```python
from build123d import *

# Parameters (mm, degrees)
F0_R            = 17.8
F0_R_2          = 7.6
F0_R_3          = 1.75
F1_DEPTH        = 10.7
F2_DEPTH        = 9.7
F2_COPIES_COUNT = 10
F3_DEPTH        = 10.7
F3_COPIES_COUNT = 10


# Not quite as in the source:
# - a pattern or mirror of a feature is missing from the dataset's text; its kind, count and spacing are read off the source's solid


with BuildPart() as f1:
    # F0 (on Top) → F1 (new body)
    with BuildSketch(Plane.XY):
        Circle(F0_R)
        Circle(F0_R_2, mode=Mode.SUBTRACT)
        with BuildLine():
            ThreePointArc((14.45, 2.5588083164), (15.4418059742, 1.4465476141), (15.8, 0))
            ThreePointArc((15.8, 0), (15.4418059742, -1.4465476141), (14.45, -2.5588083164))
            Line((14.45, -2.5588083164), (14.45, -3.5))
            Line((14.45, -3.5), (10.95, -3.5))
            Line((10.95, -3.5), (10.95, -2.5588083164))
            ThreePointArc((10.95, -2.5588083164), (9.6, 0), (10.95, 2.5588083164))
            Line((10.95, 2.5588083164), (10.95, 3.5))
            Line((10.95, 3.5), (14.45, 3.5))
            Line((14.45, 3.5), (14.45, 2.5588083164))
        make_face(mode=Mode.SUBTRACT)
        with BuildLine():
            ThreePointArc((14.45, -2.5588083164), (15.4418059742, -1.4465476141), (15.8, 0))
            ThreePointArc((15.8, 0), (15.4418059742, 1.4465476141), (14.45, 2.5588083164))
            ThreePointArc((14.45, 2.5588083164), (12.7, 3.1), (10.95, 2.5588083164))
            ThreePointArc((10.95, 2.5588083164), (9.6, 0), (10.95, -2.5588083164))
            ThreePointArc((10.95, -2.5588083164), (12.7, -3.1), (14.45, -2.5588083164))
        make_face()
        with Locations((12.7, 0)):
            Circle(F0_R_3, mode=Mode.SUBTRACT)
        with Locations((12.7, 0)):
            Circle(F0_R_3)
        with BuildLine():
            Line((14.45, -3.5), (14.45, -2.5588083164))
            ThreePointArc((14.45, -2.5588083164), (12.7, -3.1), (10.95, -2.5588083164))
            Line((10.95, -2.5588083164), (10.95, -3.5))
            Line((10.95, -3.5), (14.45, -3.5))
        make_face()
        with BuildLine():
            ThreePointArc((10.95, 2.5588083164), (12.7, 3.1), (14.45, 2.5588083164))
            Line((14.45, 2.5588083164), (14.45, 3.5))
            Line((14.45, 3.5), (10.95, 3.5))
            Line((10.95, 3.5), (10.95, 2.5588083164))
        make_face()
    extrude(amount=F1_DEPTH)

    # F0 (on Top) → F2 (cut)
    with BuildSketch(Plane.XY):
        with BuildLine():
            ThreePointArc((14.45, -2.5588083164), (15.4418059742, -1.4465476141), (15.8, 0))
            ThreePointArc((15.8, 0), (15.4418059742, 1.4465476141), (14.45, 2.5588083164))
            ThreePointArc((14.45, 2.5588083164), (12.7, 3.1), (10.95, 2.5588083164))
            ThreePointArc((10.95, 2.5588083164), (9.6, 0), (10.95, -2.5588083164))
            ThreePointArc((10.95, -2.5588083164), (12.7, -3.1), (14.45, -2.5588083164))
        make_face()
        with Locations((12.7, 0)):
            Circle(F0_R_3, mode=Mode.SUBTRACT)
        with Locations((12.7, 0)):
            Circle(F0_R_3)
    f2 = extrude(amount=F2_DEPTH, mode=Mode.SUBTRACT)

    # F2_copies: F2 ×10 about axis
    f2_copies_axis = Axis((0, 0, 0), (0, 0, 1))
    for i in range(1, F2_COPIES_COUNT):
        add(f2.rotate(f2_copies_axis, i * 360 / F2_COPIES_COUNT), mode=Mode.SUBTRACT)

    # F0 (on Top) → F3 (cut, through all)
    with BuildSketch(Plane.XY):
        with Locations((12.7, 0)):
            Circle(F0_R_3)
    f3 = extrude(amount=F3_DEPTH, mode=Mode.SUBTRACT)

    # F3_copies: F3 ×10 about axis
    f3_copies_axis = Axis((0, 0, 0), (0, 0, 1))
    for i in range(1, F3_COPIES_COUNT):
        add(f3.rotate(f3_copies_axis, i * 360 / F3_COPIES_COUNT), mode=Mode.SUBTRACT)


solid = f1.part
```
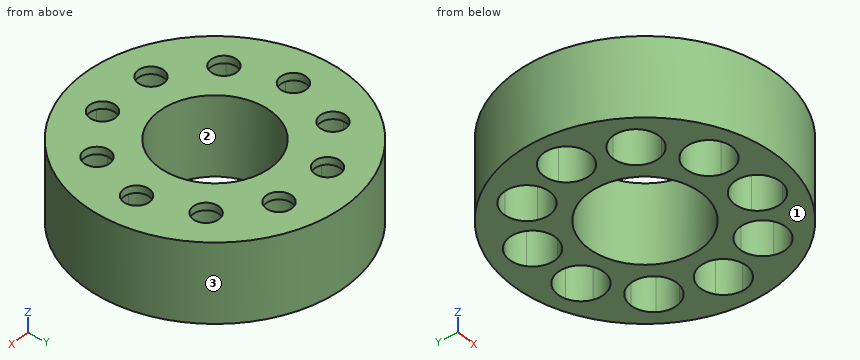
For this review, take the finished solid that the model builds, in its own axes (mm). Face numbers are marked on the shaded views. Coordinates: 2 decimals unless noted, no trailing zeros. Write each loop counter-clockwise with the first axis right and the second up, starting at its lowest first coordinate (ties: lowest second). Pieces come first, ordered by that corner, then holes. Notation, with made-up numbers: (63, 50) - (106, 50) arc R24 ccw to (106, 70) - close; hole circle Ø9 at (85.25, -4). An arc over 180 degrees is marked (long way). Answer in a Markdown table with one row per item. Add a question column.
Q1. Draft analysis for pull direction Y (two halves, no side actions). For the marked faces 1, 2 and 3, state which applies: +Y half, -Y half, draft (parallel to the pull), parting line (faces both ways), or undercut.
Q2. We need section D-D, the plane x = -4. State the section outline as (y, z) points.
Q3. We need section C-C, the plane z = 1. Count the separate pieces of the cut face and the enclosed holes in it, and give its area (3 significant figures).
Q4. We need section A-A, the plane x = 0. State the section outline as (y, z) points.
Q5. We need section B-B, the plane y = -5. State the section outline as (x, z) points, and give its area (3 significant figures).
Q6. For P1, Ø1.5, axis at x = -6.5, z = 5, coming from the -Y side; P2, Ø6, axis at y = -12, z = 4.5, coming from the -X side; P3, Ø3, axis at x = 3, y = 11.5, coming from the -Z side, all flat-tipped, find the tip position at first contact; note any pin that passes through.
Q7. For probe 1 along X at (y, z) = (6.5, 10.25); probe 2 along Y at (x, z) = (6.5, 6); probe 3 along Y at (x, z) = (-6, 8.25), list the stretches that pass through material, from the lowest coordinate up.
Answer list:
| question | item | result |
|---|---|---|
| 1 | face 1 | draft |
| 1 | face 2 | undercut |
| 1 | face 3 | parting line |
| 2 | outline | (-17.34, 0) - (-15.18, 0) - (-15.18, 9.7) - (-13.83, 9.7) - (-13.83, 10.7) - (-17.34, 10.7) - close; (-10.33, 9.7) - (-8.98, 9.7) - (-8.98, 0) - (-6.46, 0) - (-6.46, 10.7) - (-10.33, 10.7) - close; (6.46, 0) - (8.98, 0) - (8.98, 9.7) - (10.33, 9.7) - (10.33, 10.7) - (6.46, 10.7) - close; (13.83, 9.7) - (15.18, 9.7) - (15.18, 0) - (17.34, 0) - (17.34, 10.7) - (13.83, 10.7) - close |
| 3 | separate pieces | 1 |
| 3 | enclosed holes | 11 |
| 3 | area | 512 mm2 |
| 4 | outline | (-17.8, 0) - (-7.6, 0) - (-7.6, 10.7) - (-17.8, 10.7) - close; (7.6, 0) - (17.8, 0) - (17.8, 10.7) - (7.6, 10.7) - close |
| 5 | outline | (-17.08, 0) - (-12.15, 0) - (-12.15, 9.7) - (-8.39, 9.7) - (-8.39, 0) - (-5.72, 0) - (-5.72, 10.7) - (-17.08, 10.7) - close; (5.72, 0) - (8.39, 0) - (8.39, 9.7) - (12.15, 9.7) - (12.15, 0) - (17.08, 0) - (17.08, 10.7) - (5.72, 10.7) - close |
| 5 | area | 170 mm2 |
| 6 | P1 | stops at y = -16.85 |
| 6 | P2 | stops at x = -15.36 |
| 6 | P3 | stops at z = 9.7 |
| 7 | probe 1 | x = -16.57 to -11.73, -8.81 to -3.94, 3.94 to 8.81, 11.73 to 16.57 |
| 7 | probe 2 | y = -16.57 to -13.8, -10.35 to -3.94, 3.94 to 10.35, 13.8 to 16.57 |
| 7 | probe 3 | y = -16.76 to -14.38, -9.78 to -4.66, 4.66 to 9.78, 14.38 to 16.76 |
